Verification items for this drawing (mm, ordinates from the low corner). Coordinates: 2 decimals unless noted, no trailing zeros. Write each loop counter-clockwise with the first axis right and the second up, starting at its lowest first coordinate (ties: lowest second). Pieces come first, ordered by that corner, then holes. Notation, with made-up numbers: M 48,85 L 99,85 A19 ccw 99,106 Z; hole C -20,-15 d8. An arc over 180 degrees is marked long. Put each result on its own line as item: value. Start each with the question number.
1) Cross-section at C-C on z = 30. Record the cut outline in (x, y), plus the area to 3 significant figures.
2) Scan lines: line 1 along X through (y, z) = (12.75, 41); line 2 along Y through (x, z) = (12.75, 15); line 3 along Y through (x, z) = (16.75, 14). Record each from-to range of solid material in increasing order.
3) Cross-section at B-B on y = 7.5. Record the cut outline in (x, z), plus the area to 3 significant figures.
4) Gauge pin test, flat ends, axial feed: pin 1 (1.5 mm diameter, centred on y = 6.5, z = 11.5, fed in from +X); pin 2 (10 mm diameter, centred on y = 10, z = 41, fed in from -X); pin 3 (12 mm diameter, centred on x = 7, z = 35, fed in from +Y). Record the tip position at first contact, or that the pin passes through.
5) Cross-section at D-D on z = 17.5. Record the cut outline in (x, y), plus the area to 3 significant figures.
6) Cross-section at A-A on x = 17. Record the cut outline in (y, z).
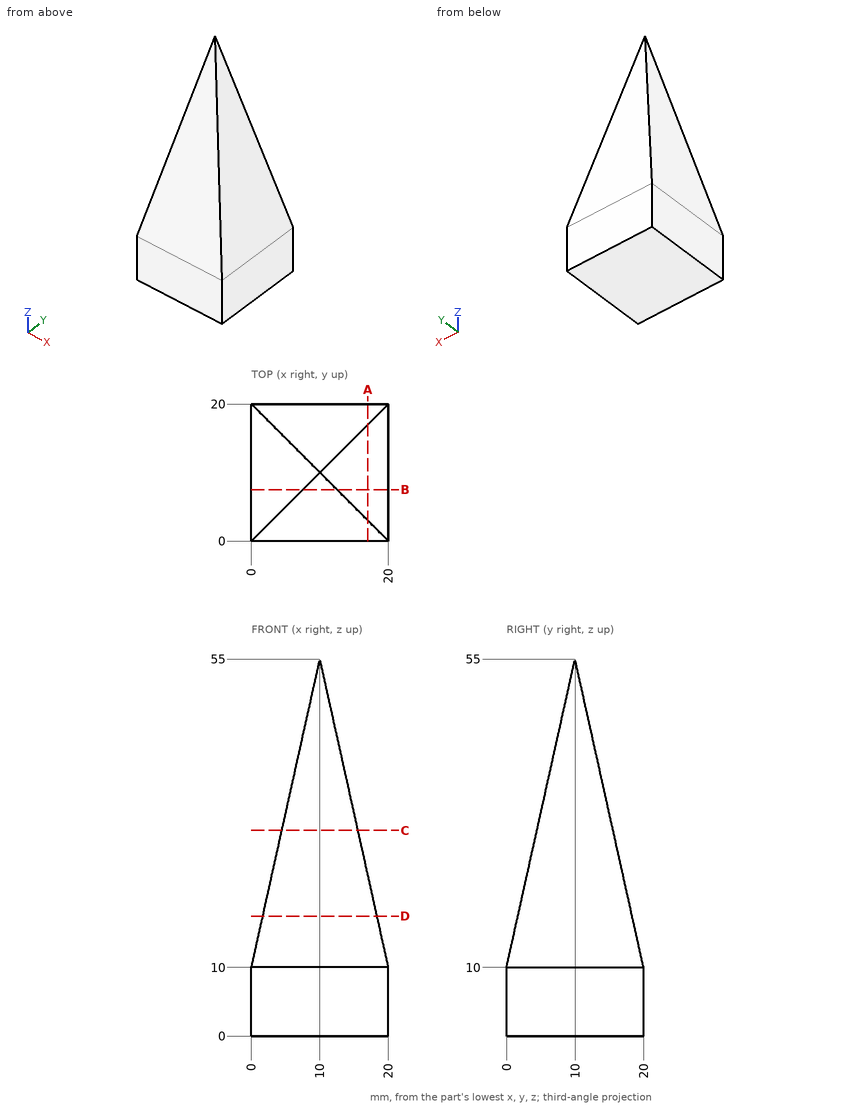
Answer key:
1. outline: M 4.44,4.44 L 15.56,4.44 L 15.56,15.56 L 4.44,15.56 Z
1. area: 123 mm²
2. line 1: x = 6.89 to 13.11
2. line 2: y = 1.11 to 18.89
2. line 3: y = 0.89 to 19.11
3. outline: M 0,0 L 20,0 L 20,10 L 12.5,43.75 L 7.5,43.75 L 0,10 Z
3. area: 622 mm²
4. pin 1: stops at x = 19.83
4. pin 2: stops at x = 5.78
4. pin 3: stops at y = 15.78
5. outline: M 1.67,1.67 L 18.33,1.67 L 18.33,18.33 L 1.67,18.33 Z
5. area: 278 mm²
6. outline: M 0,0 L 20,0 L 20,10 L 17,23.5 L 3,23.5 L 0,10 Z
